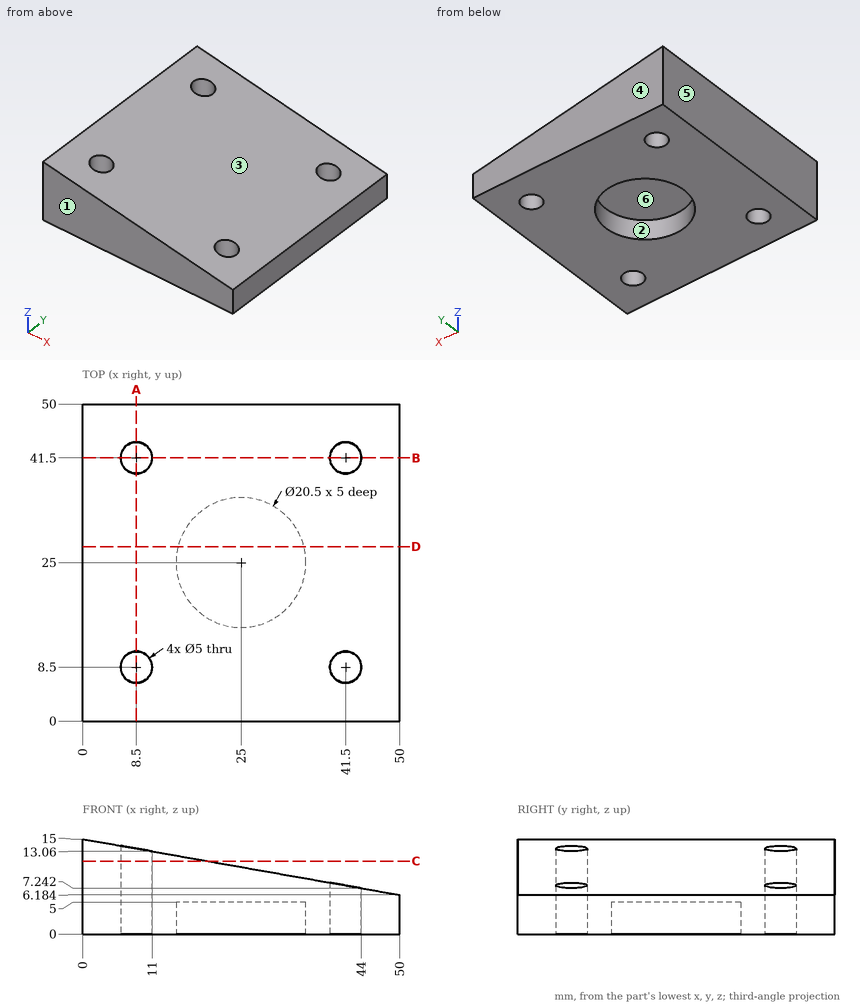
For this review, use the dimensioned drawing (mm, ordinates from the lowest corner) and the shaded views. A direction names the side the tool comes from. Coordinates: 2 decimals unless noted, no trailing zeros. Write each loop counter-clockwise with the first axis right and the second up, starting at its lowest first coordinate (ties: lowest second). Pieces come first, ordered by that corner, then holes. Notation, with made-up numbers: (26, 4) - (51, 4) arc R17 cw to (51, 31) - close; hole circle Ø11 at (49, -29). An arc over 180 degrees is marked (long way). One line per item, written item: value.
1) Add section A-A (x = 8.5). State the section outline as (y, z) points, plus the area to 3 significant figures.
Answer sheet:
outline: (0, 0) - (6, 0) - (6, 13.5) - (0, 13.5) - close; (11, 0) - (39, 0) - (39, 13.5) - (11, 13.5) - close; (44, 0) - (50, 0) - (50, 13.5) - (44, 13.5) - close
area: 540 mm2
2) Add section C-C (z = 11.5). State the section outline as (x, y) points.
Answer sheet:
outline: (0, 0) - (19.85, 0) - (19.85, 50) - (0, 50) - close; hole circle Ø5 at (8.5, 8.5); hole circle Ø5 at (8.5, 41.5)
3) Add section B-B (y = 41.5). State the section outline as (x, z) points, plus the area to 3 significant figures.
Answer sheet:
outline: (0, 0) - (6, 0) - (6, 13.94) - (0, 15) - close; (11, 0) - (39, 0) - (39, 8.12) - (11, 13.06) - close; (44, 0) - (50, 0) - (50, 6.18) - (44, 7.24) - close
area: 424 mm2
4) Mouldability with a two-part tool opening along Y and no side actions: class the marked faces 1, 2, 3 and 4 as +Y half, -Y half, draft (parallel to the pull), parting line (faces both ways), or undercut.
Answer sheet:
face 1: -Y half
face 2: undercut
face 3: draft
face 4: +Y half
5) For the marked faces 5 and 6, list the 3-axis set-ups (+Z, -Z, +X, -X, +Y, -Y) from which the entire face can be reached by the end or side of a thin tool; tool diameter is ignored.
Answer sheet:
face 5: +Z, -Z, -X, +Y, -Y
face 6: -Z
6) Insertion check: pin 1 (4.5 mm diameter, centred on x = 41.5, y = 41.5, fed in from -Z); pin 2 (12.5 mm diameter, centred on x = 25, y = 25, fed in from +Z); pin 3 (2 mm diameter, centred on x = 22.5, y = 44, fed in from +Z); pin 4 (10 mm diameter, centred on x = 24, y = 24, fed in from +Z). Each pin has a flat end and moves straight along its axis. Give the tip position at first contact, or say it passes through.
Answer sheet:
pin 1: passes through
pin 2: stops at z = 11.69
pin 3: stops at z = 11.21
pin 4: stops at z = 11.65
7) To check wall thickness, follow probe 1 along Y at (x, z) = (41.5, 2.75); probe 2 along Y at (x, z) = (25, 3.6). State the ranges of each line that lie inside material, in increasing order.
Answer sheet:
probe 1: y = 0 to 6, 11 to 39, 44 to 50
probe 2: y = 0 to 14.75, 35.25 to 50
8) Add section D-D (y = 27.5). State the section outline as (x, z) points, plus the area to 3 significant figures.
Answer sheet:
outline: (0, 0) - (15.06, 0) - (15.06, 5) - (34.94, 5) - (34.94, 0) - (50, 0) - (50, 6.18) - (0, 15) - close
area: 430 mm2
